Read the model definition and answer for the solid it produces. Units are mm, in the model's axes. A direction names the side the tool comes from. Round coordinates to 2 decimals unless told otherwise and drop trailing zeros. Order: outer loops, then holes, each group sorted by start corner. A loop starts at its lowest first (then second) coordinate and runs counter-clockwise, first axis right, second up.
from build123d import *

# Parameters (mm, degrees)
SKETCH1_W           = 5.9944
SKETCH1_H           = 5.9944
BOSS_EXTRUDE1_DEPTH = 5.9944


with BuildPart() as part:
    # Sketch1 → Boss-Extrude1 (new body)
    with BuildSketch(Plane.XY):
        with BuildLine():
            Line((384.610540851, 111.993994152), (367.537765391, 111.993994152))
            ThreePointArc((367.537765391, 111.993994152), (361.187765391, 118.343994152), (367.537765391, 124.693994152))
            Line((367.537765391, 124.693994152), (369.724153121, 124.693994152))
            ThreePointArc((369.724153121, 124.693994152), (371.520204345, 125.437942928), (372.264153121, 127.233994152))
            Line((372.264153121, 127.233994152), (372.264153121, 175.493994152))
            ThreePointArc((372.264153121, 175.493994152), (376.074153121, 179.303994152), (379.884153121, 175.493994152))
            Line((379.884153121, 175.493994152), (379.884153121, 127.233994152))
            ThreePointArc((379.884153121, 127.233994152), (380.628101897, 125.437942928), (382.424153121, 124.693994152))
            Line((382.424153121, 124.693994152), (384.610540851, 124.693994152))
            ThreePointArc((384.610540851, 124.693994152), (390.960540851, 118.343994152), (384.610540851, 111.993994152))
        make_face()
        with Locations((384.610540851, 117.991248441)):
            Rectangle(SKETCH1_W, SKETCH1_H, mode=Mode.SUBTRACT)
        with Locations((367.537765391, 117.991248441)):
            Rectangle(SKETCH1_W, SKETCH1_H, mode=Mode.SUBTRACT)
    extrude(amount=BOSS_EXTRUDE1_DEPTH)


solid = part.part
Q1. A cutting plane is placed at C-C, the plane x = 388.75. Give the vertices of the cut face in (y, z), plus the area to 3 significant figures.
Outcome:
outline: (113.53, 0) - (123.16, 0) - (123.16, 5.99) - (113.53, 5.99) - close
area: 57.7 mm2
Q2. Flat-ended cylindrical pins translate along their axes: pin 1 (1.1 mm diameter, centred on x = 383, z = 1.5, fed in from +Y); pin 2 (2 mm diameter, centred on y = 134.5, z = 3.5, fed in from -X). Find the tip coordinate at first contact, or state that the pin passes through.
Outcome:
pin 1: stops at y = 124.69
pin 2: stops at x = 372.26
Q3. For a pull along X with two mould halves and no side action, classify faces 1 (the face through (364.541, 118, 3)), 2 (the face through (376, 139, 0)), 3 (the face through (372.264, 151, 3)) as released by +X, released by -X, zero draft, split by the parting line, or undercut.
Outcome:
face 1: undercut
face 2: zero draft
face 3: released by -X
Q4. A cutting plane is placed at A-A, the plane z = 2.9. Give the vertices of the cut face in (x, y).
Outcome:
outline: (367.54, 111.99) - (384.61, 111.99) arc R6.35 ccw to (384.61, 124.69) - (382.42, 124.69) arc R2.54 cw to (379.88, 127.23) - (379.88, 175.49) arc R3.81 ccw to (372.26, 175.49) - (372.26, 127.23) arc R2.54 cw to (369.72, 124.69) - (367.54, 124.69) arc R6.35 ccw to start; hole (364.54, 114.99) - (370.53, 114.99) - (370.53, 120.99) - (364.54, 120.99) - close; hole (381.61, 114.99) - (387.61, 114.99) - (387.61, 120.99) - (381.61, 120.99) - close
Q5. For faces 4 (the face through (384, 124.694, 3)), 5 (the face through (385, 120.988, 3)), 6 (the face through (369, 124.694, 3)), determine the directions among +Z, -Z, +X, -X, +Y, -Y from which every point of the face is accessible in a straight line to the end or side of a thin tool.
Outcome:
face 4: +Z, -Z, +X, +Y
face 5: +Z, -Z
face 6: +Z, -Z, -X, +Y
Q6. A cutting plane is placed at B-B, the plane y = 135. Give the vertices of the cut face in (x, z), plus the area to 3 significant figures.
Outcome:
outline: (372.26, 0) - (379.88, 0) - (379.88, 5.99) - (372.26, 5.99) - close
area: 45.7 mm2
Q7. Straight lines are drawn through the part: probe 1 along Y at (x, z) = (368, 3.65); probe 2 along Y at (x, z) = (386.5, 1.9); probe 3 along X at (y, z) = (144, 3.3). For each, find the intervals that lie inside material, in ascending order.
Outcome:
probe 1: y = 111.99 to 114.99, 120.99 to 124.69
probe 2: y = 112.28 to 114.99, 120.99 to 124.41
probe 3: x = 372.26 to 379.88
